Part model, mm, in its own coordinate system. A direction names the side the tool comes from. Round coordinates to 2 decimals unless told otherwise and drop trailing zeros. Write each loop counter-clockwise with the first axis right and the second up, starting at its lowest first coordinate (ties: lowest second). Pieces come first, ordered by that corner, then holes.
```python
from build123d import *

# Parameters (mm, degrees)
SKETCH_1_W                         = 10
SKETCH_1_H                         = 3.8
EXTRUDE_1_DEPTH                    = 6
CUT_EXTRUDE_1_DEPTH                = 5
CUT_EXTRUDE_2_DEPTH                = 13.265398485
EXTRUDE_2_REACH                    = 14.265
CUT_EXTRUDE_3_REACH                = 14.265
SKETCH_5_W                         = 7.8
SKETCH_5_H                         = 4.1
EXTRUDE_3_REACH                    = 13.861
EXTRUDE_5_REACH                    = 14.265
SKETCH_11_W                        = 2
SKETCH_11_H                        = 3.2
SKETCH_11_W_2                      = 0.8
SKETCH_11_H_2                      = 0.8
CUT_EXTRUDE_5_DEPTH                = 0.3
SKETCH_15_R                        = 0.05
CUT_EXTRUDE_6_DEPTH                = 0.1
CHAMFER_7_SIZE                     = 0.3
PATTERN_LINEAR_2_COUNT             = 2
PATTERN_LINEAR_2_PITCH             = 2.5
EXTRUDE_START                      = -4.8
SKETCH_7_W                         = 0.6
SKETCH_7_H                         = 0.6
EXTRUDE_4_DEPTH                    = 8
CHAMFER_6_SIZE                     = 0.2
PATTERN_LINEAR_1_COUNT             = 3
PATTERN_LINEAR_1_PITCH             = 2.5
CHAMFER_7_OF_PATTERN_LINEAR_1_SIZE = 0.3
CHAMFER_6_OF_PATTERN_LINEAR_1_SIZE = 0.2
CUT_EXTRUDE_4_REACH                = 13.861
CHAMFER_5_SIZE                     = 0.3


with BuildPart() as part:
    # Эскиз1 → Бобышка-Вытянуть1 (new body)
    with BuildSketch(Plane(origin=(0, 0, 0), x_dir=(1, 0, 0), z_dir=(0, 1, 0))):
        with Locations((5, -1.9)):
            Rectangle(SKETCH_1_W, SKETCH_1_H)
    extrude(amount=EXTRUDE_1_DEPTH)

    # Эскиз2 → Вырез-Вытянуть1 (cut)
    with BuildSketch(Plane(origin=(0, 6, 0), x_dir=(1, 0, 0), z_dir=(0, 1, 0))):
        Polygon((0.5, -0.5), (9.5, -0.5), (9.5, -1.5), (8.9, -1.5), (8.9, -3.3), (1.1, -3.3), (1.1, -1.5), (0.5, -1.5), align=None)
    extrude(amount=-CUT_EXTRUDE_1_DEPTH, mode=Mode.SUBTRACT)

    # Эскиз3 → Вырез-Вытянуть2 (cut, through all)
    with BuildSketch(Plane.ZY):
        Polygon((1.8, 6), (1.8, 1.5), (2.3, 1.5), (2.7, 3.459591794), (2.7, 3.821282026), (2.4, 4.085857157), (2.4, 4.385857157), (3.1, 5.1), (3.8, 5.1), (3.8, 6), align=None)
    extrude(amount=-CUT_EXTRUDE_2_DEPTH, mode=Mode.SUBTRACT)

    # Бобышка-Вытянуть2: up to this plane
    extrude_2_end = Plane(origin=(10, 5.1, 3.1), z_dir=(0, -0.6999999999999996, 0.7141428428542854))
    # Эскиз4 → Бобышка-Вытянуть2 (add, up to the surface)
    with BuildSketch(Plane.XY.offset(3.8), mode=Mode.PRIVATE) as extrude_2_sk1:
        with BuildLine():
            Line((0.3, 5.1), (0.8, 5.1))
            ThreePointArc((0.8, 5.1), (0.55, 5.35), (0.3, 5.1))
        make_face()
    extrude_2_tool1 = split(extrude(extrude_2_sk1.sketch, amount=-EXTRUDE_2_REACH, mode=Mode.PRIVATE), bisect_by=extrude_2_end, keep=Keep.BOTH, mode=Mode.PRIVATE)
    add(extrude_2_tool1.solids().sort_by_distance((0.55, 5.206103, 3.8))[0])

    # Эскиз5 → Вырез-Вытянуть3 (cut, up to next)
    with BuildSketch(Plane.XY.offset(3.8), mode=Mode.PRIVATE) as cut_extrude_3_sk1:
        with Locations((5, 3.05)):
            Rectangle(SKETCH_5_W, SKETCH_5_H)
    cut_extrude_3_tool1 = extrude(cut_extrude_3_sk1.sketch, amount=-CUT_EXTRUDE_3_REACH, mode=Mode.PRIVATE) & part.part
    add(cut_extrude_3_tool1.solids().sort_by_distance((5, 3.05, 3.8))[0], mode=Mode.SUBTRACT)

    # Эскиз6 → Бобышка-Вытянуть3 (add, up to next)
    with BuildSketch(Plane(origin=(0.5, 0, 0), x_dir=(0, 0, -1), z_dir=(1, 0, 0)), mode=Mode.PRIVATE) as extrude_3_sk1:
        Polygon((-2.9, 1), (-2.27, 1.5), (-0.5, 1.5), (-0.5, 1), align=None)
    extrude_3_tool1 = extrude(extrude_3_sk1.sketch, amount=EXTRUDE_3_REACH, mode=Mode.PRIVATE) - part.part
    add(extrude_3_tool1.solids().sort_by_distance((0.5, 1.23741, 1.550432))[0])

    # Эскиз9 → Бобышка-Вытянуть5 (add, up to next)
    with BuildSketch(Plane(origin=(0, 6, 0), x_dir=(1, 0, 0), z_dir=(0, 1, 0)), mode=Mode.PRIVATE) as extrude_5_sk1:
        Polygon((3.45, -0.5), (3.75, -0.928444402), (4.05, -0.5), align=None)
    extrude_5_tool1 = extrude(extrude_5_sk1.sketch, amount=-EXTRUDE_5_REACH, mode=Mode.PRIVATE) - part.part
    extrude_5 = extrude_5_tool1.solids().sort_by_distance((3.75, 6, 0.642815))[0]
    add(extrude_5)

    # Эскиз11 → Вырез-Вытянуть5 (cut)
    with BuildSketch(Plane.XZ):
        with Locations((2.5, 1.6)):
            Rectangle(SKETCH_11_W, SKETCH_11_H)
        with Locations((2.5, 1.6)):
            Rectangle(SKETCH_11_W_2, SKETCH_11_H_2, mode=Mode.SUBTRACT)
    cut_extrude_5 = extrude(amount=-CUT_EXTRUDE_5_DEPTH, mode=Mode.SUBTRACT)

    # Эскиз15 → Вырез-Вытянуть6 (cut)
    with BuildSketch(Plane.XZ):
        with Locations(Location((2.5, 1.6, 0), (0, 0, 270))):
            Circle(SKETCH_15_R)
    extrude(amount=-CUT_EXTRUDE_6_DEPTH, mode=Mode.SUBTRACT)

    # Фаска7
    chamfer_7_edges = [part.edges().sort_by_distance(p)[0] for p in [
        (1.5, 0.3, 1.6),
        (2.5, 0.3, 3.2),
        (3.5, 0.3, 1.6),
        (2.9, 0.3, 1.6),
        (2.5, 0.3, 2),
        (2.1, 0.3, 1.6),
        (2.5, 0.3, 1.2),
    ]]
    chamfer(chamfer_7_edges, length=CHAMFER_7_SIZE - 0.0001)  # a hair under: the kernel refuses the full size

    # Линейный массив2: Бобышка-Вытянуть5 ×2
    with Locations(*[(i * PATTERN_LINEAR_2_PITCH, 0, 0) for i in range(1, PATTERN_LINEAR_2_COUNT)]):
        add(extrude_5)

    # Эскиз7 → Бобышка-Вытянуть4 (add)
    with BuildSketch(Plane.XZ.offset(EXTRUDE_START)):
        with Locations((2.5, 1.6)):
            Rectangle(SKETCH_7_W, SKETCH_7_H)
    extrude_4 = extrude(amount=EXTRUDE_4_DEPTH)

    # Фаска6
    chamfer_6_edges = [part.edges().sort_by_distance(p)[0] for p in [
        (2.8, 4.8, 1.6),
        (2.5, 4.8, 1.9),
        (2.2, 4.8, 1.6),
        (2.5, 4.8, 1.3),
        (2.8, -3.2, 1.6),
        (2.5, -3.2, 1.9),
        (2.2, -3.2, 1.6),
        (2.5, -3.2, 1.3),
    ]]
    chamfer(chamfer_6_edges, length=CHAMFER_6_SIZE)

    # Линейный массив1: Вырез-Вытянуть5, Бобышка-Вытянуть4 ×3
    with Locations(*[(i * PATTERN_LINEAR_1_PITCH, 0, 0) for i in range(1, PATTERN_LINEAR_1_COUNT)]):
        add(cut_extrude_5, mode=Mode.SUBTRACT)
        add(extrude_4)

    # Фаска7 of Линейный массив1
    chamfer_7_of_pattern_linear_1_edges = [part.edges().sort_by_distance(p)[0] for p in [
        (4, 0.3, 1.6),
        (5, 0.3, 3.2),
        (6, 0.3, 1.6),
        (5.4, 0.3, 1.6),
        (5, 0.3, 2),
        (4.6, 0.3, 1.6),
        (5, 0.3, 1.2),
        (6.5, 0.3, 1.6),
        (7.5, 0.3, 3.2),
        (8.5, 0.3, 1.6),
        (7.9, 0.3, 1.6),
        (7.5, 0.3, 2),
        (7.1, 0.3, 1.6),
        (7.5, 0.3, 1.2),
    ]]
    chamfer(chamfer_7_of_pattern_linear_1_edges, length=CHAMFER_7_OF_PATTERN_LINEAR_1_SIZE - 0.0001)  # a hair under: the kernel refuses the full size

    # Фаска6 of Линейный массив1
    chamfer_6_of_pattern_linear_1_edges = [part.edges().sort_by_distance(p)[0] for p in [
        (5.3, 4.8, 1.6),
        (5, 4.8, 1.9),
        (4.7, 4.8, 1.6),
        (5, 4.8, 1.3),
        (5.3, -3.2, 1.6),
        (5, -3.2, 1.9),
        (4.7, -3.2, 1.6),
        (5, -3.2, 1.3),
        (7.8, 4.8, 1.6),
        (7.5, 4.8, 1.9),
        (7.2, 4.8, 1.6),
        (7.5, 4.8, 1.3),
        (7.8, -3.2, 1.6),
        (7.5, -3.2, 1.9),
        (7.2, -3.2, 1.6),
        (7.5, -3.2, 1.3),
    ]]
    chamfer(chamfer_6_of_pattern_linear_1_edges, length=CHAMFER_6_OF_PATTERN_LINEAR_1_SIZE)

    # Вырез-Вытянуть4: up to this face of the body (flat: up to its plane)
    cut_extrude_4_end = Plane(part.part.faces().sort_by_distance((9.5, 3.75, 1))[0])
    # Эскиз10 → Вырез-Вытянуть4 (cut, up to the picked face)
    with BuildSketch(Plane(origin=(0.5, 0, 0), x_dir=(0, 0, -1), z_dir=(1, 0, 0)), mode=Mode.PRIVATE) as cut_extrude_4_sk1:
        Polygon((-1, 6), (-0.2, 6), (-1, 5.2), (-1, 5.1), (-1.8, 5.1), (-1.8, 6), align=None)
    cut_extrude_4_tool1 = split(extrude(cut_extrude_4_sk1.sketch, amount=CUT_EXTRUDE_4_REACH, mode=Mode.PRIVATE), bisect_by=cut_extrude_4_end, keep=Keep.BOTH, mode=Mode.PRIVATE)
    add(cut_extrude_4_tool1.solids().sort_by(Axis((0.5, 5.60641, 1.194872), (1, 0, 0)))[0], mode=Mode.SUBTRACT)

    # Фаска5
    chamfer_5_edges = [part.edges().sort_by_distance(p)[0] for p in [
        (9.5, 6, 1),
        (0.5, 6, 1),
    ]]
    chamfer(chamfer_5_edges, length=CHAMFER_5_SIZE)


solid = part.part
```
Q1. Mould opens along Z. For faces 4 (the flat face through (4.93, 0.85, 3.8)), 5 (the flat face through (1.1, 3, 3)), 6 (the flat face through (5, 4, 0.5)) say: +Z half, -Z half, draft (parallel to the pull), parting line (faces both ways), or undercut.
Values follow:
face 4: +Z half
face 5: draft
face 6: undercut
Q2. Drop flat-ended pins along their axis: pin 1 (0.7 mm diameter, centred on y = -1.5, z = 1.5, fed in from -X); pin 2 (0.5 mm diameter, centred on x = 5, y = -2, fed in from +Z). Give the stop position or say it passes through.
Values follow:
pin 1: stops at x = 2.2
pin 2: stops at z = 1.9
Q3. Cut at A-A on y = 3.25. State how many separate pieces and enclosed holes the cut face has, plus the area to 3 significant figures.
Values follow:
separate pieces: 6
enclosed holes: 0
area: 10.5 mm2
Q4. Wall check: L1, parallel to X at y = -1, z = 1.85; L2, parallel to X at y = 2.75, z = 1.25; L3, parallel to X at y = 0.25, z = 0.4. Give the ranges that are in metal, low to high.
Values follow:
L1: x = 2.2 to 2.8, 4.7 to 5.3, 7.2 to 7.8
L2: x = 0 to 0.5, 9.5 to 10
L3: x = 0 to 1.75, 3.25 to 4.25, 5.75 to 6.75, 8.25 to 10
Q5. Which spindle directions (+Z, -Z, +X, -X, +Y, -Y) get a long thin tool onto all of the face, cutting with end or side? Do faces 1 (the flat face through (0.54, 2.47, 2.5)), 2 (the flat face through (8.9, 3, 3)), 3 (the flat face through (0.5, 4, 1)). Say none if no direction does.
Values follow:
face 1: +X, -X
face 2: +Z, +Y
face 3: +Y
Q6. Cut at B-B on y = 1.25. Write the cut outline in (x, z) (3 decimals), plus the area to 3 significant figures.
Values follow:
outline: (0, 0) - (10, 0) - (10, 3.8) - (8.9, 3.8) - (8.9, 2.585) - (1.1, 2.585) - (1.1, 3.8) - (0, 3.8) - close
area: 28.5 mm2
